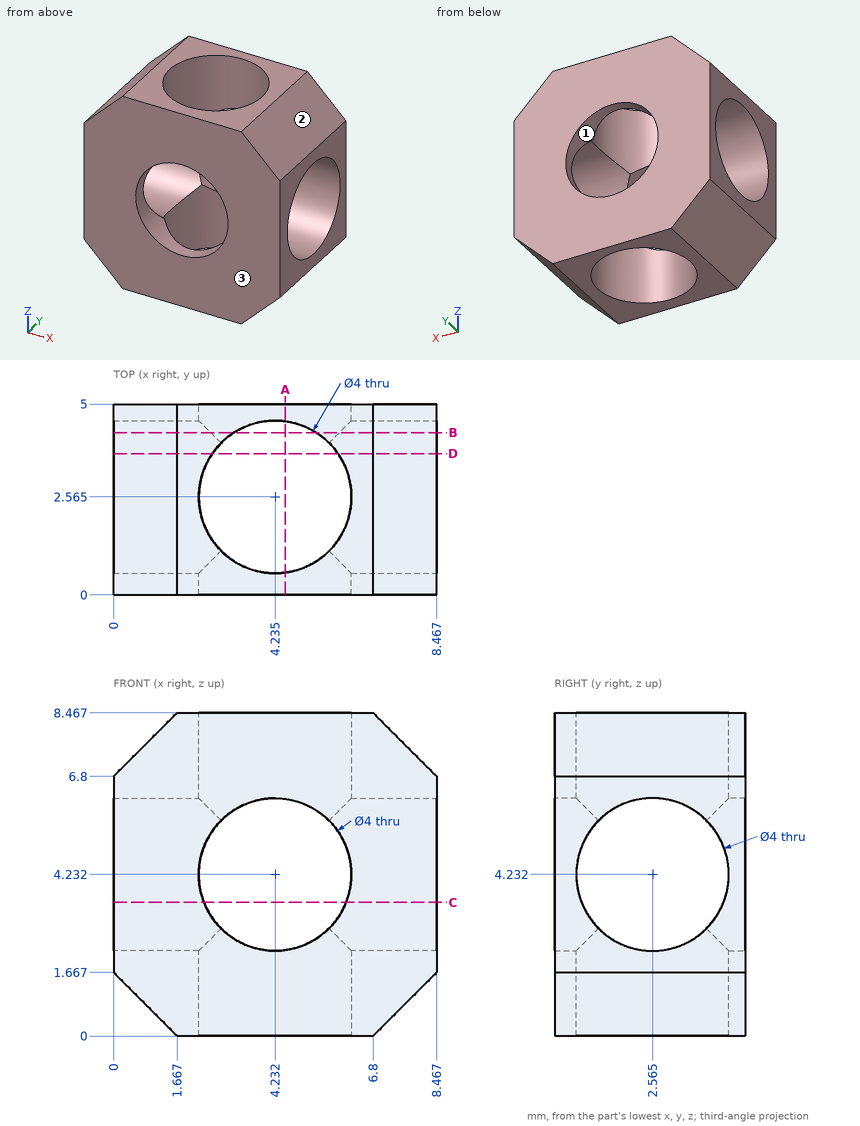
Geometry: see drawing. Coordinates: mm, zero at the bounding-box minimum. Coordinates: 2 decimals unless noted, no trailing zeros. Loops run counter-clockwise (first coordinate to the right, second up) from the corner with the lowest first, then second, coordinate; pieces in that order, holes last. Notation, with made-up numbers: M 36.25,-13.5 L 83.25,-13.5 A32 ccw 83.25,21.5 Z; hole C -13.75,77.5 d8. An arc over 180 degrees is marked long. Answer in a Markdown table with one row per item.
1. Section A-A, the plane x = 4.5. Output: boundary loops of the cut face in (y, z).
Response:
| item | result |
|---|---|
| outline | M 0,0 L 0.58,0 L 0.58,2.25 L 0,2.25 Z; M 0,6.21 L 0.58,6.21 L 0.58,8.47 L 0,8.47 Z; M 4.55,0 L 5,0 L 5,2.25 L 4.55,2.25 Z; M 4.55,6.21 L 5,6.21 L 5,8.47 L 4.55,8.47 Z |
2. Section C-C, the plane z = 3.5. Output: boundary loops of the cut face in (x, y).
Response:
| item | result |
|---|---|
| outline | M 0,0 L 2.37,0 L 2.37,0.7 L 0,0.7 Z; M 0,4.43 L 2.37,4.43 L 2.37,5 L 0,5 Z; M 6.09,0 L 8.47,0 L 8.47,0.7 L 6.09,0.7 Z; M 6.09,4.43 L 8.47,4.43 L 8.47,5 L 6.09,5 Z |
3. Section B-B, the plane y = 4.25. Output: boundary loops of the cut face in (x, z) (1 decimal).
Response:
| item | result |
|---|---|
| outline | M 0,1.7 L 1.7,0 L 3.2,0 L 3.2,2.5 A2 cw 2.5,3.2 L 0,3.2 Z; M 0,5.3 L 2.5,5.3 A2 cw 3.2,5.9 L 3.2,8.5 L 1.7,8.5 L 0,6.8 Z; M 5.3,0 L 6.8,0 L 8.5,1.7 L 8.5,3.2 L 5.9,3.2 A2 cw 5.3,2.5 Z; M 5.3,5.9 A2 cw 5.9,5.3 L 8.5,5.3 L 8.5,6.8 L 6.8,8.5 L 5.3,8.5 Z |
4. First-contact query: pin 1 (1 mm diameter, centred on x = 1, y = 3, fed in from -Z). Flat tip, straight axial feed; report the tip coordinate or a pass-through.
Response:
| item | result |
|---|---|
| pin 1 | stops at z = 0.17 |
5. Draft query along X for the marked faces 1, 2 and 3. Return one class per face: pulls with the +X half, pulls with the -X half, needs draft (parallel to the pull), parting line crosses it, or undercut.
Response:
| item | result |
|---|---|
| face 1 | undercut |
| face 2 | pulls with the +X half |
| face 3 | needs draft |
6. Material intervals for line 1 (Y direction, x = 7.75, z = 4.5); line 2 (Y direction, x = 3.5, z = 2) (1 decimal); line 3 (X direction, y = 0.85, z = 1.5) (1 decimal), sorted ascending.
Response:
| item | result |
|---|---|
| line 1 | y = 0 to 0.58, 4.55 to 5 |
| line 2 | y = 0 to 0.7, 4.4 to 5 |
| line 3 | x = 0.2 to 3.2, 5.3 to 8.3 |
7. Section D-D, the plane y = 3.7. Output: boundary loops of the cut face in (x, z) (1 decimal), then the cut area to 3 significant figures.
Response:
| item | result |
|---|---|
| outline | M 0,1.7 L 1.7,0 L 2.6,0 L 2.6,2.6 L 0,2.6 Z; M 0,5.9 L 2.6,5.9 L 2.6,8.5 L 1.7,8.5 L 0,6.8 Z; M 5.9,0 L 6.8,0 L 8.5,1.7 L 8.5,2.6 L 5.9,2.6 Z; M 5.9,5.9 L 8.5,5.9 L 8.5,6.8 L 6.8,8.5 L 5.9,8.5 Z |
| area | 21.2 mm2 |
